Could you check a few things on this model? Use its own coordinates, in mm. A direction names the side the tool comes from. Give positions to 0.01 mm unless a question says otherwise; leave off trailing zeros. Order: outer loops, then holes, each group sorted by start corner. A loop starts at its lowest first (then second) coordinate and runs counter-clockwise, first axis right, second up.
(1) Will these pins go through, and if not, where does the flat tip stop? pin 1 (4 mm diameter, centred on x = -12, z = -14, fed in from -Y); pin 2 (1 mm diameter, centred on x = -7.5, y = 13, fed in from -Z); pin 3 (5 mm diameter, centred on y = -0.5, z = -12.5, fed in from -X).
(2) Imagine slicing it at A-A, the plane z = -5.75. Write out the boundary of the cut face in (x, y), then the cut area to 3 significant figures.
(3) Imagine slicing it at D-D, the plane y = 3.5. Write out the boundary of the cut face in (x, z), then the cut area to 3 significant figures.
(4) Imagine slicing it at B-B, the plane x = -6.5. Write out the boundary of the cut face in (y, z).
(5) If we mould it in two halves opening along Z, with no side actions, what happens to faces 5 (the flat face through (-16, 13, -14.284)), 6 (the flat face through (-13.353, 13, -17)), 7 (the flat face through (-9, 12.6, -10))? For each: released by +Z, released by -Z, zero draft, split by the parting line, or undercut.
(6) If I drill on probe 1 along Y at (x, z) = (-6, -13.5); probe 2 along Y at (x, z) = (-7.5, -6); probe 3 along Y at (x, z) = (-10.75, -14.5), over which ranges is the centre line in solid material (lowest first)?
(7) On a 3-axis mill with a long thin cutter (end or side, diameter ignored), from which of +Z, -Z, +X, -X, +Y, -Y can I reach the whole of each face in a straight line? I mean faces 1 (the flat face through (-13, -2, -9.784)), 2 (the flat face through (-9, 6, -3.284)), 3 (the cylindrical face through (-6.803, -1.521, -7.594)), 4 (the flat face through (-13.353, 3, -5)). Say none if no direction works.
(8) Imagine slicing it at C-C, the plane x = -13.75. Write out the boundary of the cut face in (y, z).
from build123d import *

# Parameters (mm, degrees)
ESQUISSE1_W             = 9
ESQUISSE1_H             = 9
BOSS_EXTRU_1_DEPTH      = 3
ENL_V_MAT_EXTRU_1_DEPTH = 20.782165931
ESQUISSE3_W             = 9
ESQUISSE3_H             = 18.3
BOSS_EXTRU_3_DEPTH      = 2
ESQUISSE4_W             = 9
ESQUISSE4_H             = 3.7
BOSS_EXTRU_4_DEPTH      = 8
BOSS_EXTRU_6_DEPTH      = 3
BOSS_EXTRU_8_DEPTH      = 1
CONG_2_R                = 4
CONG_3_R                = 2
ESQUISSE7_R             = 1.329968568
ENL_V_MAT_EXTRU_2_DEPTH = 1
CONG_4_R                = 1


with BuildPart() as part:
    # Esquisse1 → Boss.-Extru.1 (new body)
    with BuildSketch(Plane(origin=(0, 0, 0), x_dir=(1, 0, 0), z_dir=(0, 1, 0))):
        with Locations((-8.852843945, 9.784104714)):
            Rectangle(ESQUISSE1_W, ESQUISSE1_H)
    extrude(amount=-BOSS_EXTRU_1_DEPTH)

    # Esquisse2 → Enlèv. mat.-Extru.1 (cut, through all)
    with BuildSketch(Plane.XZ.offset(3)):
        with BuildLine():
            Line((-8.852843945, -12.784104714), (-8.852843945, -14.284104714))
            Line((-8.852843945, -14.284104714), (-13.352843945, -14.284104714))
            Line((-13.352843945, -14.284104714), (-13.352843945, -9.784104714))
            Line((-13.352843945, -9.784104714), (-11.852843945, -9.784104714))
            ThreePointArc((-11.852843945, -9.784104714), (-6.731523602, -7.66278437), (-8.852843945, -12.784104714))
        make_face()
    extrude(amount=-ENL_V_MAT_EXTRU_1_DEPTH, mode=Mode.SUBTRACT)

    # Esquisse3 → Boss.-Extru.3 (add)
    with BuildSketch(Plane.XY.offset(-5.284104714)):
        with Locations((-8.852843945, 6.15)):
            Rectangle(ESQUISSE3_W, ESQUISSE3_H)
    extrude(amount=BOSS_EXTRU_3_DEPTH)

    # Esquisse4 → Boss.-Extru.4 (add)
    with BuildSketch(Plane(origin=(0, 0, -5.284104714), x_dir=(-1, 0, 0), z_dir=(0, 0, -1))):
        with Locations((8.852843945, 13.45)):
            Rectangle(ESQUISSE4_W, ESQUISSE4_H)
    extrude(amount=BOSS_EXTRU_4_DEPTH)

    # Esquisse8 → Boss.-Extru.6 (add)
    with BuildSketch(Plane(origin=(0, 15.3, 0), x_dir=(1, 0, 0), z_dir=(0, 1, 0))):
        Polygon((-18.352843945, 3.284104714), (-4.352843945, 3.284104714), (-4.352843945, 19.284104714), (-13.352843945, 19.284104714), (-13.352843945, 14.284104714), (-18.352843945, 14.284104714), align=None)
    extrude(amount=-BOSS_EXTRU_6_DEPTH)

    # Esquisse9 → Boss.-Extru.8 (add)
    with BuildSketch(Plane(origin=(0, 15.3, 0), x_dir=(1, 0, 0), z_dir=(0, 1, 0))):
        Polygon((-18.352843945, 16.284104714), (-18.352843945, 3.284104714), (-4.352843945, 3.284104714), (-4.352843945, 19.284104714), (-15.352843945, 19.284104714), (-15.352843945, 16.284104714), align=None)
    extrude(amount=-BOSS_EXTRU_8_DEPTH)

    # Congé2
    cong_2_edges = [part.edges().sort_by_distance(p)[0] for p in [
        (-18.352843945, 13.8, -3.284104714),
        (-4.352843945, 13.8, -19.284104714),
    ]]
    fillet(cong_2_edges, radius=CONG_2_R)

    # Congé3
    cong_3_edges = [part.edges().sort_by_distance(p)[0] for p in [
        (-15.352843945, 14.8, -16.284104714),
    ]]
    fillet(cong_3_edges, radius=CONG_3_R)

    # Esquisse7 → Enlèv. mat.-Extru.2 (cut)
    with BuildSketch(Plane.XZ.offset(-11.6)):
        with Locations(Location((-8.852843945, -9.784104714, 0), (0, 0, 270))):
            Circle(ESQUISSE7_R)
    extrude(amount=-ENL_V_MAT_EXTRU_2_DEPTH, mode=Mode.SUBTRACT)

    # Congé4
    cong_4_edges = [part.edges().sort_by_distance(p)[0] for p in [
        (-15.352843945, 14.8, -19.284104714),
        (-18.352843945, 14.8, -16.284104714),
    ]]
    fillet(cong_4_edges, radius=CONG_4_R - 0.0001)  # a hair under: the kernel refuses the full size


solid = part.part
Answer block:
1. pin 1: stops at y = 11.6
1. pin 2: stops at z = -19.27
1. pin 3: stops at x = -8.85
2. outline: (-18.05, 12.3) - (-13.35, 12.3) - (-13.35, 11.6) - (-4.35, 11.6) - (-4.35, 15.3) - (-18.05, 15.3) - close; (-13.35, -3) - (-4.35, -3) - (-4.35, 0) - (-13.35, 0) - close
2. area: 74.4 mm2
3. outline: (-13.35, -5.28) - (-4.35, -5.28) - (-4.35, -3.28) - (-13.35, -3.28) - close
3. area: 18.0 mm2
4. outline: (-3, -14.28) - (0, -14.28) - (0, -11.65) - (-3, -11.65) - close; (-3, -7.92) - (0, -7.92) - (0, -5.28) - (11.6, -5.28) - (11.6, -13.28) - (12.3, -13.28) - (12.3, -18.83) - (15.3, -18.83) - (15.3, -3.28) - (-3, -3.28) - close
5. face 5: released by -Z
5. face 6: zero draft
5. face 7: undercut
6. probe 1: y = -3 to 0, 12.3 to 15.3
6. probe 2: y = -3 to 0, 11.6 to 15.3
6. probe 3: y = 12.3 to 15.3
7. face 1: -Z, -X, -Y
7. face 2: +Z, +X, -X, +Y, -Y
7. face 3: -Y
7. face 4: +Z, -Z, -X, -Y
8. outline: (12.3, -14.28) - (14.3, -14.28) - (14.3, -19.28) - (15.3, -19.28) - (15.3, -3.28) - (12.3, -3.28) - close
